Part model, mm, in its own coordinate system. A direction names the side the tool comes from. Give positions to 0.01 mm unless a question says otherwise; leave off trailing zeros. Write each loop counter-clockwise with the first axis right and the second up, starting at its lowest first coordinate (ties: lowest second). Pieces come first, ordered by that corner, then holes. Notation, with made-up numbers: (-2.5, -40) - (8.5, -40) arc R13 ccw to (8.5, -24) - close; hole circle Ø8 at (-35.75, 49.25). An arc over 180 degrees is marked (long way). Answer in a Markdown table with one row per item. Add a question column.
1. Pull direction Y, two halves, no side cores. Call faces 6 (the flat face through (-21, 11.95, 3)), 7 (the flat face through (-12.2, 5, 3)), 8 (the flat face through (2.5, -9, 2)), 9 (the flat face through (-25, -6.15, 2)): released by +Y, released by -Y, zero draft, split by the parting line, or undercut.
2. Drop flat-ended pins along their axis: pin 1 Ø1.5 at (y, z) = (21.5, 2) entering from -X; pin 2 Ø1.5 at (x, z) = (26, 2.5) entering from +Y; pin 3 Ø1.5 at (y, z) = (-9.5, 1.5) entering from +X. Give the stop position or say it passes through.
3. Band-saw the part on A-A on x = -16. Write the cut outline in (y, z).
4. Band-saw the part on B-B on y = 19.5. Write the cut outline in (x, z), plus the area to 3 significant figures.
5. Probe line 1 along X through (y, z) = (-7, 3.2); line 2 along X through (y, z) = (7, 2.25); line 3 along Y through (x, z) = (-16.5, 4.3). List the from-to ranges inside material, lowest first.
6. Which spindle directions (+Z, -Z, +X, -X, +Y, -Y) get a long thin tool onto all of the face, cutting with end or side? Do faces 1 (the flat face through (55, -6.15, 2)), 2 (the flat face through (-52.5, 21, 2)), 3 (the flat face through (25, 18.45, 2)), 4 (the flat face through (-52.5, -9, 2)), 5 (the flat face through (-2.5, -9, 2)). Say none if no direction does.
7. Band-saw the part on C-C on y = 0.5. Write the cut outline in (x, z).
```python
from build123d import *

# Parameters (mm, degrees)
SKETCH1_W           = 116
SKETCH1_H           = 12.3
BOSS_EXTRUDE1_DEPTH = 5
SKETCH2_W           = 5
SKETCH2_H           = 5
BOSS_EXTRUDE2_DEPTH = 5
SKETCH3_W           = 17
SKETCH3_H           = 13.5
CUT_EXTRUDE1_DEPTH  = 6


with BuildPart() as part:
    # Sketch1 → Boss-Extrude1 (new body)
    with BuildSketch(Plane.XY):
        Rectangle(SKETCH1_W, SKETCH1_H)
    extrude(amount=BOSS_EXTRUDE1_DEPTH)

    # Sketch2 → Boss-Extrude2 (add)
    with BuildSketch(Plane.XZ.offset(6.15)):
        with Locations((-50, 2.5)):
            Rectangle(SKETCH2_W, SKETCH2_H)
        with Locations((0, 2.5)):
            Rectangle(SKETCH2_W, SKETCH2_H)
        with Locations((50, 2.5)):
            Rectangle(SKETCH2_W, SKETCH2_H)
    extrude(amount=BOSS_EXTRUDE2_DEPTH)

    # Mirror1: part across plane


with BuildPart() as part_1:
    add(part.part)
    add(part.part.mirror(Plane(origin=(-58, 6.15, 5), x_dir=(0, 0, 1), z_dir=(0, -1, 0))))

    # Sketch3 → Cut-Extrude1 (cut, through all)
    with BuildSketch(Plane.XY.offset(5)):
        with Locations((-20.7, 5.2)):
            Rectangle(SKETCH3_W, SKETCH3_H)
    extrude(amount=-CUT_EXTRUDE1_DEPTH, mode=Mode.SUBTRACT)


solid = part_1.part
```
Values:
| question | item | result |
|---|---|---|
| 1 | face 6 | undercut |
| 1 | face 7 | undercut |
| 1 | face 8 | zero draft |
| 1 | face 9 | released by -Y |
| 2 | pin 1 | stops at x = -52.5 |
| 2 | pin 2 | stops at y = 18.45 |
| 2 | pin 3 | stops at x = 52.5 |
| 3 | outline | (-6.15, 0) - (-1.55, 0) - (-1.55, 5) - (-6.15, 5) - close; (11.95, 0) - (18.45, 0) - (18.45, 5) - (11.95, 5) - close |
| 4 | outline | (-52.5, 0) - (-47.5, 0) - (-47.5, 5) - (-52.5, 5) - close; (-2.5, 0) - (2.5, 0) - (2.5, 5) - (-2.5, 5) - close; (47.5, 0) - (52.5, 0) - (52.5, 5) - (47.5, 5) - close |
| 4 | area | 75.0 mm² |
| 5 | line 1 | x = -52.5 to -47.5, -2.5 to 2.5, 47.5 to 52.5 |
| 5 | line 2 | x = -58 to -29.2, -12.2 to 58 |
| 5 | line 3 | y = -6.15 to -1.55, 11.95 to 18.45 |
| 6 | face 1 | +Z, -Z, +X, -Y |
| 6 | face 2 | +Z, -Z, -X, +Y |
| 6 | face 3 | +Z, -Z, +Y |
| 6 | face 4 | +Z, -Z, -X, -Y |
| 6 | face 5 | +Z, -Z, -Y |
| 7 | outline | (-58, 0) - (-29.2, 0) - (-29.2, 5) - (-58, 5) - close; (-12.2, 0) - (58, 0) - (58, 5) - (-12.2, 5) - close |
